Geometry: final body of the model. Coordinates: model frame, mm. Coordinates: 2 decimals unless noted, no trailing zeros. Order: outer loops, then holes, each group sorted by start corner. A loop starts at its lowest first (then second) coordinate and runs counter-clockwise, first axis right, second up. Notation, with made-up numbers: (-22.5, -23) -> (14.5, -23) arc R14 cw to (14.5, -5) -> close; hole circle Ø8 at (-30.5, 24). An arc over 180 degrees is marked (long way). Answer in a Markdown table with one row per item. Add a question column.
1) Ray query, line 1 (Y direction, x = 0.25, z = 0.55); line 2 (Z direction, x = -0.05, y = -6.75); line 3 (Y direction, x = 0.8, z = -1.45). Return the intervals inside material, ascending. Write a range as from..to.
2) Section query D-D on y = -5.5. Return the cut outline in (x, z), then the cut area to 3 significant figures.
3) Section query A-A on x = 0. Return the cut outline in (y, z), then the cut area to 3 significant figures.
4) Contact query for flat-ended pins moving along their axis: P1, Ø2, axis at x = 0.5, y = -1.5, coming from the -Z side; P2, Ø0.8, axis at x = 0, z = 0, coming from the +Y side. Output: stop coordinate, or through.
5) Section query B-B on z = 0. Return the cut outline in (x, y), then the cut area to 3 significant figures.
6) Section query C-C on y = 1. Return the cut outline in (x, z), then the cut area to 3 significant figures.
7) Pull-direction query (X, two-part tool) for faces 1 (the face through (-1.5, -4.68, -0.07)), 2 (the face through (-1.2, 0, -1.2)), 3 (the face through (0, 1.25, 0)); classes: +X half, -X half, draft (parallel to the pull), parting line (faces both ways), or undercut.
Autodesk Inventor part; units mm, degrees
ref_plane "YZ Plane" through (0, 0, 0) normal (1, 0, 0) x (0, 1, 0)
ref_plane "XZ Plane" through (0, 0, 0) normal (0, 1, 0) x (-1, 0, 0)
ref_plane "XY Plane" through (0, 0, 0) normal (0, 0, 1) x (1, 0, 0)
sketch "Sketch1" plane through (0, 0, 0) normal (0, 1, 0) x (-1, 0, 0)
  circle A0 centre (0, 0) radius 2.7
  dimension "headDiameter" = 5.4
extrude "Extrusion1" add sketch "Sketch1" along normal blind 2
sketch "Sketch2" plane through (0, 2, 0) normal (0, 1, 0) x (1, 0, 0)
  line L0 (0.5, -2.7) -> (-0.5, -2.7)
  line L1 (-0.5, -2.7) -> (-0.5, 2.7)
  line L2 (-0.5, 2.7) -> (0.5, 2.7)
  line L3 (0.5, 2.7) -> (0.5, -2.7)
  line L4 (0.5, -2.7) -> (-0.5, 2.7) construction
  line L5 (-0.5, -2.7) -> (0.5, 2.7) construction
  point P0 (0, 0)
  dimension "d3" = 1
  dimension "d4" = 5.4
extrude "Extrusion2" cut sketch "Sketch2" against normal blind 0.75
sketch "Sketch3" plane through (0, 0, 0) normal (0, -1, 0) x (1, 0, 0)
  circle A0 centre (0, 0) radius 1.5
  dimension "d7" = 3
extrude "Extrusion3" add sketch "Sketch3" along normal blind 10
chamfer "Chamfer1" distance 0.5 angle 45 1 edges at (-1.5, -10, 0)
fillet "Fillet1" radius 0.5 3 edges at (-2.0785, 2, 1.7234) (-2.0785, 2, -1.7234) (2.7, 2, 0)
equation "\"d4\" = headDiameter"
properties part number "machineScrew3x10" material "Stainless Steel"
Result:
| question | item | result |
|---|---|---|
| 1 | line 1 | -10..1.25 |
| 1 | line 2 | -1.5..1.5 |
| 1 | line 3 | 0..2 |
| 2 | outline | circle Ø3 at (0, 0) |
| 2 | area | 7.07 mm2 |
| 3 | outline | (-10, -1) -> (-9.5, -1.5) -> (0, -1.5) -> (0, -2.7) -> (1.25, -2.7) -> (1.25, 2.7) -> (0, 2.7) -> (0, 1.5) -> (-9.5, 1.5) -> (-10, 1) -> close |
| 3 | area | 36.5 mm2 |
| 4 | P1 | z = -1.5 |
| 4 | P2 | y = 1.25 |
| 5 | outline | (-2.7, 0) -> (-1.5, 0) -> (-1.5, -9.5) -> (-1, -10) -> (1, -10) -> (1.5, -9.5) -> (1.5, 0) -> (2.7, 0) -> (2.7, 1.5) arc R0.5 ccw to (2.2, 2) -> (0.5, 2) -> (0.5, 1.25) -> (-0.5, 1.25) -> (-0.5, 2) -> (-2.2, 2) arc R0.5 ccw to (-2.7, 1.5) -> close |
| 5 | area | 39.7 mm2 |
| 6 | outline | circle Ø5.4 at (0, 0) |
| 6 | area | 22.9 mm2 |
| 7 | face 1 | parting line |
| 7 | face 2 | draft |
| 7 | face 3 | undercut |
